Autodesk Inventor part; units mm, degrees
ref_plane "YZ Plane" through (0, 0, 0) normal (1, 0, 0) x (0, 1, 0)
ref_plane "XZ Plane" through (0, 0, 0) normal (0, 1, 0) x (-1, 0, 0)
ref_plane "XY Plane" through (0, 0, 0) normal (0, 0, 1) x (1, 0, 0)
sketch "スケッチ1" plane through (0, 0, 0) normal (0, 0, 1) x (1, 0, 0)
  line L0 (0, 0) -> (40, 0)
  line L1 (40, 0) -> (40, 60)
  line L2 (40, 60) -> (0, 60)
  line L3 (0, 60) -> (0, 0)
  line L4 (0, 10) -> (40, 10) construction
  circle A0 centre (10, 10) radius 2
  circle A1 centre (30, 10) radius 2
  line L5 (20, 60) -> (20, 40) construction
  circle A2 centre (20, 40) radius 4.1
  dimension "d0" = 10
  dimension "d1" = 10
  dimension "d2" = 10
  dimension "d3" = 40
  dimension "d4" = 4
  dimension "d5" = 8.2
  dimension "d6" = 40
  dimension "d7" = 20
extrude "押し出し1" add sketch "スケッチ1" along normal blind 10
sketch "スケッチ2" plane through (0, 0, 10) normal (0, 0, 1) x (1, 0, 0)
  line L0 (40, 60) -> (0, 60) construction
  line L1 (20, 60) -> (20, 0) construction
  line L2 (0, 0) -> (40, 0) construction
  line L3 (0, 60) -> (8, 60)
  line L4 (8, 60) -> (8, 50)
  line L5 (8, 50) -> (0, 50)
  line L6 (0, 50) -> (0, 60)
  line L7 (40, 0) -> (40, 60)
  line L8 (40, 60) -> (32, 60)
  line L9 (32, 60) -> (32, 50)
  line L10 (32, 50) -> (40, 50)
  line L11 (40, 50) -> (40, 60)
  line L12 (19, 80) -> (21, 80)
  line L13 (21, 80) -> (21, 40)
  line L14 (21, 40) -> (19, 40)
  line L15 (19, 40) -> (19, 80)
  line L16 (19, 80) -> (21, 40) construction
  line L17 (21, 80) -> (19, 40) construction
  circle A0 centre (20, 40) radius 4.1
  dimension "d11" = 10
  dimension "d12" = 8
  dimension "d13" = 2
extrude "押し出し2" cut sketch "スケッチ2" against normal blind 10 contours L3 L4 L5 L6 | L10 L9 L8 L7 | L12 L13 A0 L15 | A0 L13 L14 L15 picked at (19.8879, 41.3621)
sketch "スケッチ3" plane through (0, 0, 0) normal (-1, 0, 0) x (0, 0, 1)
  line L0 (0, 0) -> (10, 0) construction
  line L1 (5, 0) -> (5, 59.7235) construction
  circle A0 centre (5, 55) radius 2
  line L2 (10, 60) -> (0, 60) construction
  dimension "d16" = 5
  dimension "d17" = 4
extrude "押し出し3" cut sketch "スケッチ3" against normal through all
fillet "フィレット1" radius 2 4 edges at (0, 0, 5) (40, 0, 5) (40, 50, 5) (0, 50, 5)
properties part number "ガイド輪マウント"
Here's how the part is built. I have some questions about the finished solid (model axes, mm). A direction names the side the tool comes from. Give positions to 0.01 mm unless a question says otherwise; leave off trailing zeros. Loops run counter-clockwise (first coordinate to the right, second up) from the corner with the lowest first, then second, coordinate; pieces in that order, holes last. Notation, with made-up numbers: (62, -21.5) -> (92, -21.5) arc R30 ccw to (92, 8.5) -> close; hole circle Ø2 at (-2.75, 13.25). An arc over 180 degrees is marked (long way). Use one line per item in the form item = value. Start each with the question number.
1) Thinking about a two-plate mould opening in Y: for faces 1 (the face through (14, 60, 5)), 2 (the face through (0.57, 0.6, 5.07)), 3 (the face through (31.908, 9.399, 4.93)), which applies, +Y half, -Y half, draft (parallel to the pull), parting line (faces both ways), or undercut?
2) Imagine slicing it at A-A (z = 1.5). Please give me the cut outline in (x, y).
3) Imagine slicing it at B-B (z = 5). Please give me the cut outline in (x, y), then the cut area to 3 significant figures.
4) For P1, Ø3.5, axis at x = 10, y = 10, coming from the -Z side; P2, Ø3, axis at x = 34, z = 5.5, coming from the +Y side; P3, Ø4.5, axis at y = 55, z = 5, coming from the +X side, each with a flat end and sliding along its axis, tell me the tip position at first contact or that it passes through.
5) Imagine slicing it at D-D (y = 40). Please give me the cut outline in (x, z).
6) Imagine slicing it at C-C (y = 55). Please give me the cut outline in (x, z), then the cut area to 3 significant figures.
7) Which directions (+Z, -Z, +X, -X, +Y, -Y) give clear straight access to the entire face, cutting with the end or side of a thin tool? Please do faces 4 (the face through (19, 52, 5)), 5 (the face through (32, 57.3, 5.1)), 6 (the face through (8, 57.3, 5.1)).
8) Please list where these lines run through material, in increasing order: line 1 along X through (y, z) = (51.5, 2.5); line 2 along Y through (x, z) = (30, 6.5); line 3 along X through (y, z) = (40, 2.5).
Check values:
q1.face_1 = +Y half
q1.face_2 = -Y half
q1.face_3 = undercut
q2.outline = (0, 2) arc R2 ccw to (2, 0) -> (38, 0) arc R2 ccw to (40, 2) -> (40, 48) arc R2 ccw to (38, 50) -> (32, 50) -> (32, 60) -> (21, 60) -> (21, 43.98) arc R4.1 cw (long way) to (19, 43.98) -> (19, 60) -> (8, 60) -> (8, 50) -> (2, 50) arc R2 ccw to (0, 48) -> close; hole circle Ø4 at (10, 10); hole circle Ø4 at (30, 10)
q3.outline = (0, 2) arc R2 ccw to (2, 0) -> (38, 0) arc R2 ccw to (40, 2) -> (40, 48) arc R2 ccw to (38, 50) -> (32, 50) -> (32, 53) -> (21, 53) -> (21, 43.98) arc R4.1 cw (long way) to (19, 43.98) -> (19, 53) -> (8, 53) -> (8, 50) -> (2, 50) arc R2 ccw to (0, 48) -> close; (8, 57) -> (19, 57) -> (19, 60) -> (8, 60) -> close; (21, 57) -> (32, 57) -> (32, 60) -> (21, 60) -> close; hole circle Ø4 at (10, 10); hole circle Ø4 at (30, 10)
q3.area = 2,040 mm^2
q4.P1 = through
q4.P2 = 50
q4.P3 = 32
q5.outline = (0, 0) -> (15.9, 0) -> (15.9, 10) -> (0, 10) -> close; (24.1, 0) -> (40, 0) -> (40, 10) -> (24.1, 10) -> close
q6.outline = (8, 0) -> (19, 0) -> (19, 3) -> (8, 3) -> close; (8, 7) -> (19, 7) -> (19, 10) -> (8, 10) -> close; (21, 0) -> (32, 0) -> (32, 3) -> (21, 3) -> close; (21, 7) -> (32, 7) -> (32, 10) -> (21, 10) -> close
q6.area = 132 mm^2
q7.face_4 = +Z, -Z, +Y
q7.face_5 = +Z, -Z, +X, +Y
q7.face_6 = +Z, -Z, -X, +Y
q8.line_1 = 8 to 19, 21 to 32
q8.line_2 = 0 to 8, 12 to 53.68, 56.32 to 60
q8.line_3 = 0 to 15.9, 24.1 to 40
